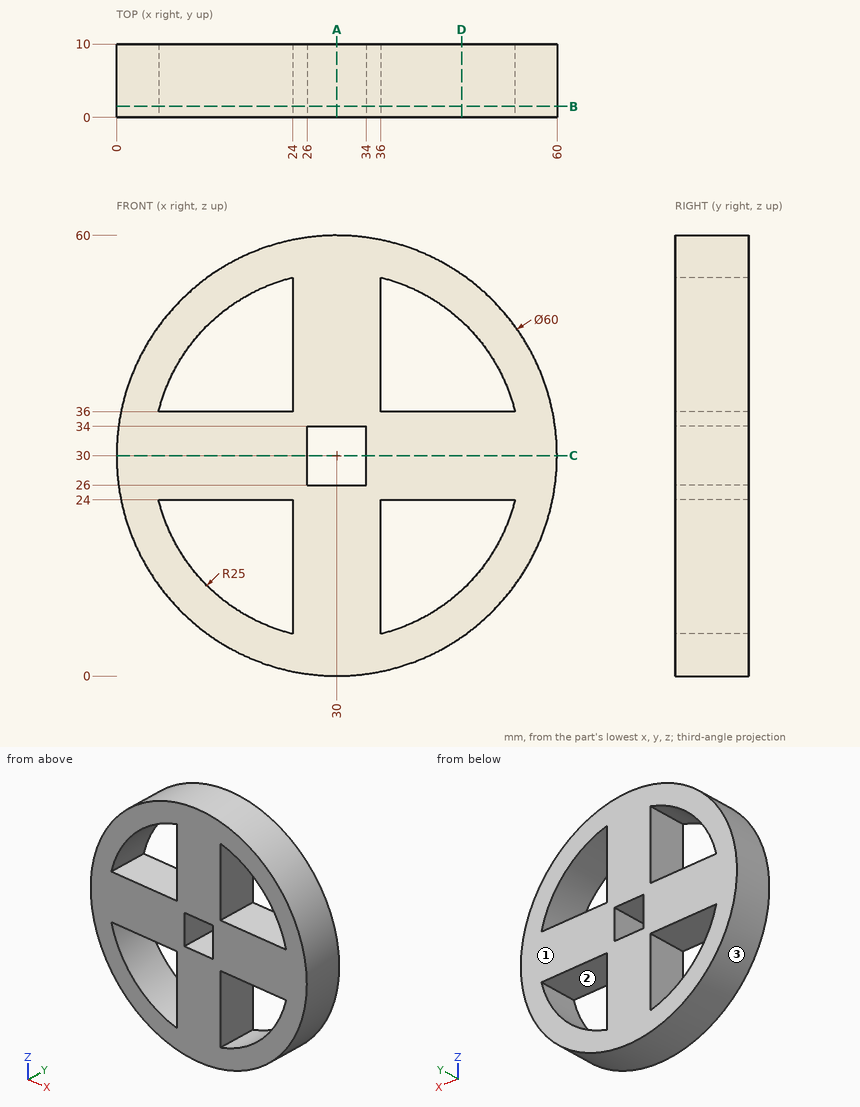
Design review of the part shown in the three views and the two pictorial views. Dimensions are in mm from the part's minimum x, y and z. Round coordinates to 2 decimals unless told otherwise and drop trailing zeros. Order: outer loops, then holes, each group sorted by start corner. A loop starts at its lowest first (then second) coordinate and runs counter-clockwise, first axis right, second up. Notation, with made-up numbers: M -28,8.25 L -23,8.25 A26 cw -23,31.25 Z; hole C 53.5,45 d5. An arc over 180 degrees is marked long. Put each result on its own line as item: value.
Q1. Consider section A-A (x = 30). State the section outline as (y, z) points, and give its area (3 significant figures).
Reported:
outline: M 0,0 L 10,0 L 10,26 L 0,26 Z; M 0,34 L 10,34 L 10,60 L 0,60 Z
area: 520 mm²
Q2. Consider section C-C (z = 30). State the section outline as (x, y) points, and give its area (3 significant figures).
Reported:
outline: M 0,0 L 26,0 L 26,10 L 0,10 Z; M 34,0 L 60,0 L 60,10 L 34,10 Z
area: 520 mm²
Q3. Consider section D-D (x = 47). State the section outline as (y, z) points, and give its area (3 significant figures).
Reported:
outline: M 0,5.28 L 10,5.28 L 10,11.67 L 0,11.67 Z; M 0,24 L 10,24 L 10,36 L 0,36 Z; M 0,48.33 L 10,48.33 L 10,54.72 L 0,54.72 Z
area: 248 mm²
Q4. Insertion check: pin 1 Ø5 at (x, y) = (6.5, 5.5) entering from +Z; pin 2 Ø5 at (y, z) = (6.5, 18) entering from -X; pin 3 Ø3 at (x, y) = (48.5, 7.5) entering from -Z. Each pin has a flat end and moves straight along its axis. Give the tip position at first contact, or say it passes through.
Reported:
pin 1: z = 51.42
pin 2: x = 1.54
pin 3: z = 5.28
Q5. Consider section B-B (y = 1.5). State the section outline as (x, z) points, and give its area (3 significant figures).
Reported:
outline: C 30,30 d60; hole M 5.73,24 A25 ccw 24,5.73 L 24,24 Z; hole M 5.73,36 L 24,36 L 24,54.27 A25 ccw Z; hole M 26,26 L 34,26 L 34,34 L 26,34 Z; hole M 36,5.73 A25 ccw 54.27,24 L 36,24 Z; hole M 36,36 L 54.27,36 A25 ccw 36,54.27 Z
area: 1,840 mm²
Q6. Draft analysis for pull direction Z (two halves, no side actions). For the marked faces 1, 2 and 3, state which applies: released by +Z, released by -Z, zero draft, split by the parting line, or undercut.
Reported:
face 1: zero draft
face 2: undercut
face 3: split by the parting line
Q7. To check wall thickness, follow line 1 (Z direction, x = 7, y = 6.5); line 2 (X direction, y = 9.25, z = 45). State the ranges of each line that lie inside material, in increasing order.
Reported:
line 1: 10.74 to 20.2, 24 to 36, 39.8 to 49.26
line 2: 4.02 to 10, 24 to 36, 50 to 55.98
